from build123d import *

# Parameters (mm, degrees)
HOLE_WIZARD_M31_D           = 3.4
HOLE_WIZARD_M31_CSINK_D     = 6.3
HOLE_WIZARD_M31_CSINK_ANGLE = 90


with BuildPart() as part:
    # Эскиз1 → Повернуть1 (revolve)
    with BuildSketch(Plane(origin=(0, 0, 0), x_dir=(0, 0, -1), z_dir=(1, 0, 0))):
        Polygon((22, 1), (22, 4), (0, 4), (0, 0), (19.5, 0), align=None)
    revolve(axis=Axis((0, 0, 0), (0, 1, 0)))

    # Зенковка для винта с полупотайной головкой M31 (through all)
    with Locations(Plane(origin=(0, 4, 0), x_dir=(1, 0, 0), z_dir=(0, 1, 0))):
        with Locations((6.5, 11.258330249), (13, 0), (6.5, -11.258330249), (-6.5, -11.258330249), (-13, 0), (-6.5, 11.258330249)):
            CounterSinkHole(HOLE_WIZARD_M31_D / 2, HOLE_WIZARD_M31_CSINK_D / 2, counter_sink_angle=HOLE_WIZARD_M31_CSINK_ANGLE)


solid = part.part
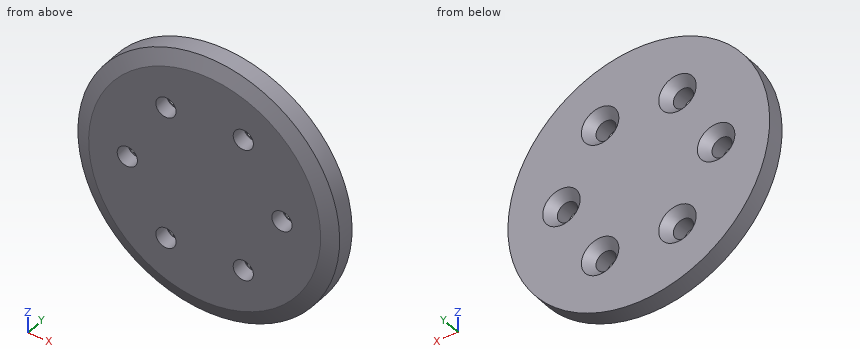
Design review of the part built by this model. Coordinates are the model's own, in mm. Give positions to 0.01 mm unless a question says otherwise; leave off trailing zeros. Write each loop counter-clockwise with the first axis right and the second up, starting at its lowest first coordinate (ties: lowest second). Pieces come first, ordered by that corner, then holes. Notation, with made-up numbers: M 49.5,8.5 L 97.5,8.5 A19 ccw 97.5,40.5 Z; hole C -39,24.5 d5. An arc over 180 degrees is marked long. Return JSON: item names as keys, results as strings. Group by question number.
Item 1: Clearance check with flat-ended pins moving along their axes: pin 1 Ø1 at (x, y) = (-15.5, 2.5) entering from +Z; pin 2 Ø2.5 at (x, z) = (6.5, 11.26) entering from -Y; pin 3 Ø1.5 at (y, z) = (1, -12.5) entering from +X; pin 4 Ø1 at (y, z) = (2, 4.5) entering from +X. State where each tip first meets the part, or that it passes through.
Item 2: Take a section at A-A (z = 0). Give the boundary of the cut face in (x, y), plus the area to 3 significant figures.
Item 3: Take a section at C-C (x = -6.5). Count the separate pieces of the cut face and the enclosed holes in it, plus the area to 3 significant figures.
Item 4: Take a section at B-B (y = 1.9). Give the boundary of the cut face in (x, z), plus the area to 3 significant figures.
Item 5: Wall thickness on line 1 along Z through (x, y) = (-6.5, 1.5); line 2 along X through (y, z) = (1.5, -10.5); line 3 along X through (y, z) = (0.25, -1.5): over which ranges is each line inside the solid? List them lowest first.
Return value:
{
 "1": {"pin 1": "stops at z = 16.09", "pin 2": "passes through", "pin 3": "stops at x = 18.6", "pin 4": "stops at x = 21.63"},
 "2": {"outline": "M -22,1 L -19.5,0 L -14.7,0 L -14.7,2.55 L -16.15,4 L -22,4 Z; M -11.3,0 L 11.3,0 L 11.3,2.55 L 9.85,4 L -9.85,4 L -11.3,2.55 Z; M 14.7,0 L 19.5,0 L 22,1 L 22,4 L 16.15,4 L 14.7,2.55 Z", "area": "142 mm2"},
 "3": {"separate pieces": "3", "enclosed holes": "0", "area": "134 mm2"},
 "4": {"outline": "C 0,0 d44; hole C -13,0 d3.4; hole C -6.5,-11.26 d3.4; hole C -6.5,11.26 d3.4; hole C 6.5,-11.26 d3.4; hole C 6.5,11.26 d3.4; hole C 13,0 d3.4", "area": "1,470 mm2"},
 "5": {"line 1": "z = -21.02 to -12.96, -9.56 to 9.56, 12.96 to 21.02", "line 2": "x = -19.33 to -8.02, -4.98 to 4.98, 8.02 to 19.33", "line 3": "x = -20.07 to -13.8, -12.2 to 12.2, 13.8 to 20.07"}
}
